from build123d import *

# Parameters (mm, degrees)
SKETCH1_R           = 53.2765
BOSS_EXTRUDE1_DEPTH = 21.971
SKETCH3_R           = 51.689
CUT_EXTRUDE2_DEPTH  = 18.796
CUT_EXTRUDE7_DEPTH  = 18.796
SKETCH7_R           = 6.477
BOSS_EXTRUDE3_DEPTH = 10.9855


with BuildPart() as part:
    # Sketch1 → Boss-Extrude1 (new body)
    with BuildSketch(Plane(origin=(0, 0, 0), x_dir=(1, 0, 0), z_dir=(0, 1, 0))):
        Circle(SKETCH1_R)
    extrude(amount=BOSS_EXTRUDE1_DEPTH)

    # Sketch3 → Cut-Extrude2 (cut)
    with BuildSketch(Plane(origin=(0, 21.971, 0), x_dir=(1, 0, 0), z_dir=(0, 1, 0))):
        Circle(SKETCH3_R)
    extrude(amount=-CUT_EXTRUDE2_DEPTH, mode=Mode.SUBTRACT)

    # Sketch6 → Cut-Extrude7 (cut)
    with BuildSketch(Plane(origin=(0, 21.971, 0), x_dir=(1, 0, 0), z_dir=(0, 1, 0))):
        with BuildLine():
            Line((23.516654444, 46.029552298), (23.788647289, 47.670595889))
            ThreePointArc((23.788647289, 47.670595889), (17.831858769, 50.203687764), (11.611838625, 51.995679205))
            Line((11.611838625, 51.995679205), (11.333405616, 50.431206987))
            ThreePointArc((11.333405616, 50.431206987), (17.563465277, 48.613551696), (23.516654444, 46.029552298))
        make_face()
    extrude(amount=-CUT_EXTRUDE7_DEPTH, mode=Mode.SUBTRACT)

    # Sketch7 → Boss-Extrude3 (add)
    with BuildSketch(Plane.XZ):
        with BuildLine():
            ThreePointArc((50.217200735, -17.793768644), (87.757, 0), (50.217200735, 17.793768644))
            ThreePointArc((50.217200735, 17.793768644), (53.2765, 0), (50.217200735, -17.793768644))
        make_face()
        with Locations((64.77, 0)):
            Circle(SKETCH7_R, mode=Mode.SUBTRACT)
        with BuildLine():
            ThreePointArc((-50.217200735, 17.793768644), (-87.757, 0), (-50.217200735, -17.793768644))
            ThreePointArc((-50.217200735, -17.793768644), (-53.2765, 0), (-50.217200735, 17.793768644))
        make_face()
        with Locations((-64.77, 0)):
            Circle(SKETCH7_R, mode=Mode.SUBTRACT)
    extrude(amount=-BOSS_EXTRUDE3_DEPTH)


solid = part.part
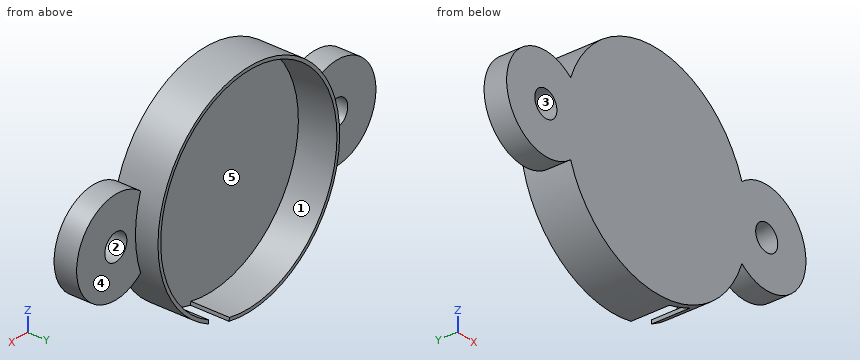
Can you work these out from the model? Positions are in its coordinate system, mm. Face numbers are marked on the shaded views. A direction names the side the tool comes from. Round coordinates to 2 decimals unless told otherwise and drop trailing zeros. Loops run counter-clockwise (first coordinate to the right, second up) from the corner with the lowest first, then second, coordinate; pieces in that order, holes last. Notation, with made-up numbers: (6.25, 73) - (51.25, 73) arc R6 cw to (51.25, 78) - close; hole circle Ø11 at (11, 39.5). An arc over 180 degrees is marked (long way). Use CSV: the item, a comma, the result in double quotes. Start each with the question number.
1) For the marked faces 1 and 2, which set-ups out of +Z, -Z, +X, -X, +Y, -Y let a thin tool reach every point of the face, with its end or its side?
2) If we section it at D-D on y = 8.25: Write out the boundary of the cut face in (x, z), plus the area to 3 significant figures.
3) If we section it at A-A on x = -64.77: Write out the boundary of the cut face in (y, z), plus the area to 3 significant figures.
4) Please list where these lines run through material, in increasing order: probe 1 along Z at (x, y) = (0, 9.5); probe 2 along Y at (x, z) = (62.5, -18.5); probe 3 along Y at (x, z) = (-21, -20) (3 decimals). Write a range as [from, to].
5) For pin 1 Ø2 at (x, y) = (-6, 17) entering from -Z; pin 2 Ø12 at (y, z) = (15, -13.5) entering from -X; pin 3 Ø8 at (y, z) = (6.5, -22) entering from +X, each with a flat end and sliding along its axis, tell me the tip position at first contact or that it passes through.
6) We'd pull the mould along X, two halves only. Please class the marked faces 3, 4 and 5: released by +X, released by -X, zero draft, split by the parting line, or undercut.
7) If we section it at B-B on z = 0: Write out the boundary of the cut face in (x, y) (1 decimal).
8) If we section it at C-C on x = 0: Write out the boundary of the cut face in (y, z) (1 decimal), plus the area to 3 significant figures.
Geometry results:
1,face 1,"+Y"
1,face 2,"+Y, -Y"
2,outline,"(-50.22, -17.79) arc R53.28 ccw to (11.61, -52) - (11.33, -50.43) arc R51.69 cw (long way) to (23.52, -46.03) - (23.79, -47.67) arc R53.28 ccw to (50.22, -17.79) arc R22.99 ccw (long way) to (50.22, 17.79) arc R53.28 ccw to (-50.22, 17.79) arc R22.99 ccw (long way) to start; hole circle Ø12.95 at (-64.77, 0); hole circle Ø12.95 at (64.77, 0)"
2,area,"3,000 mm2"
3,outline,"(0, -22.99) - (10.99, -22.99) - (10.99, -6.48) - (0, -6.48) - close; (0, 6.48) - (10.99, 6.48) - (10.99, 22.99) - (0, 22.99) - close"
3,area,"363 mm2"
4,probe 1,"z = [-53.28, -51.69], [51.69, 53.28]"
4,probe 2,"y = [0, 10.99]"
4,probe 3,"y = [0, 3.175]"
5,pin 1,"stops at z = -53.04"
5,pin 2,"stops at x = -85.9"
5,pin 3,"stops at x = 79.07"
6,face 3,"undercut"
6,face 4,"zero draft"
6,face 5,"undercut"
7,outline,"(-87.8, 0) - (-71.2, 0) - (-71.2, 11) - (-87.8, 11) - close; (-58.3, 0) - (58.3, 0) - (58.3, 11) - (53.3, 11) - (53.3, 22) - (51.7, 22) - (51.7, 3.2) - (-51.7, 3.2) - (-51.7, 22) - (-53.3, 22) - (-53.3, 11) - (-58.3, 11) - close; (71.2, 0) - (87.8, 0) - (87.8, 11) - (71.2, 11) - close"
8,outline,"(0, -53.3) - (22, -53.3) - (22, -51.7) - (3.2, -51.7) - (3.2, 51.7) - (22, 51.7) - (22, 53.3) - (0, 53.3) - close"
8,area,"398 mm2"
